The model under review builds one solid part; all positions refer to its coordinate system, in mm. Face numbers are marked on the shaded views. Give positions to 0.01 mm unless a question says otherwise; leave off trailing zeros. Order: outer loops, then holes, each group sorted by start corner. A loop starts at its lowest first (then second) coordinate and runs counter-clockwise, first axis right, second up. Notation, with made-up numbers: M 32,-6 L 61,-6 A20 cw 61,19 Z; hole C 45.25,81.5 d3. An arc over 180 degrees is marked long. One line per question, with ' | ' between items. Start each with the question number.
1. Insertion check: P1, Ø3, axis at y = -2, z = -8, coming from the +X side; P2, Ø6, axis at x = -37.5, z = 2.5, coming from the +Y side; P3, Ø10, axis at x = -41.5, y = -1.5, coming from the +Z side; P4, Ø1.5, axis at x = -38.5, z = 3, coming from the -Y side. Each pin has a flat end and moves straight along its axis. Give the tip position at first contact, or say it passes through.
2. Wall thickness on L1, parallel to Y at x = -2.15, z = 0; L2, parallel to Y at x = -34, z = 0; L3, parallel to X at y = 3.25, z = 5: over which ranges is each line inside the solid? List them lowest first.
3. The part is to be moulded in two halves that separate along Y. For the marked faces 1, 2 and 3, say which applies: +Y half, -Y half, draft (parallel to the pull), parting line (faces both ways), or undercut.
4. We need section A-A on x = -37.5. Write out the cut boundary in (y, z), then the cut area to 3 significant figures.
```python
from build123d import *


with BuildPart() as part:
    # Sketch1 → Base-Revolve (revolve)
    with BuildSketch(Plane.XY, mode=Mode.PRIVATE) as base_revolve_sk:
        with BuildLine():
            Line((0, 8), (0, 6.794144144))
            ThreePointArc((0, 6.794144144), (0.796034843, 5.848666431), (-0.1025, 5))
            Line((-0.1025, 5), (-43, 5))
            Line((-43, 5), (-43, 10))
            ThreePointArc((-43, 10), (-46.218807741, 6.847700542), (-47.4, 2.5))
            Line((-47.4, 2.5), (-47.4, 0))
            Line((-47.4, 0), (-5.783270352, 0))
            Line((-5.783270352, 0), (-3.5, 3.8))
            Line((-3.5, 3.8), (0, 3.8))
            ThreePointArc((0, 3.8), (2, 5.9), (0, 8))
        make_face()
    revolve(base_revolve_sk.sketch.rotate(Axis((40.376928104, 0, 0), (-1, 0, 0)), 90), axis=Axis((40.376928104, 0, 0), (-1, 0, 0)))


solid = part.part
```
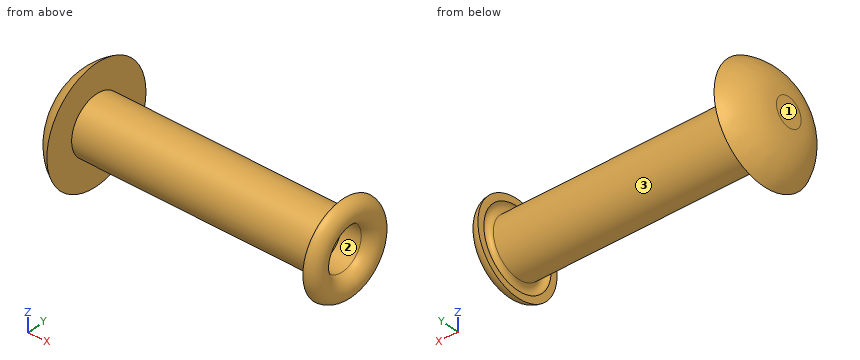
Entries:
1) P1: stops at x = 1.82 | P2: stops at y = 5 | P3: stops at z = 10 | P4: stops at y = -4.47
2) L1: y = -5 to -3.8, 3.8 to 5 | L2: y = -5 to 5 | L3: x = -46.67 to -43, 0.8 to 2
3) face 1: draft | face 2: undercut | face 3: parting line
4) outline: C 0,0 d10 | area: 78.5 mm^2
